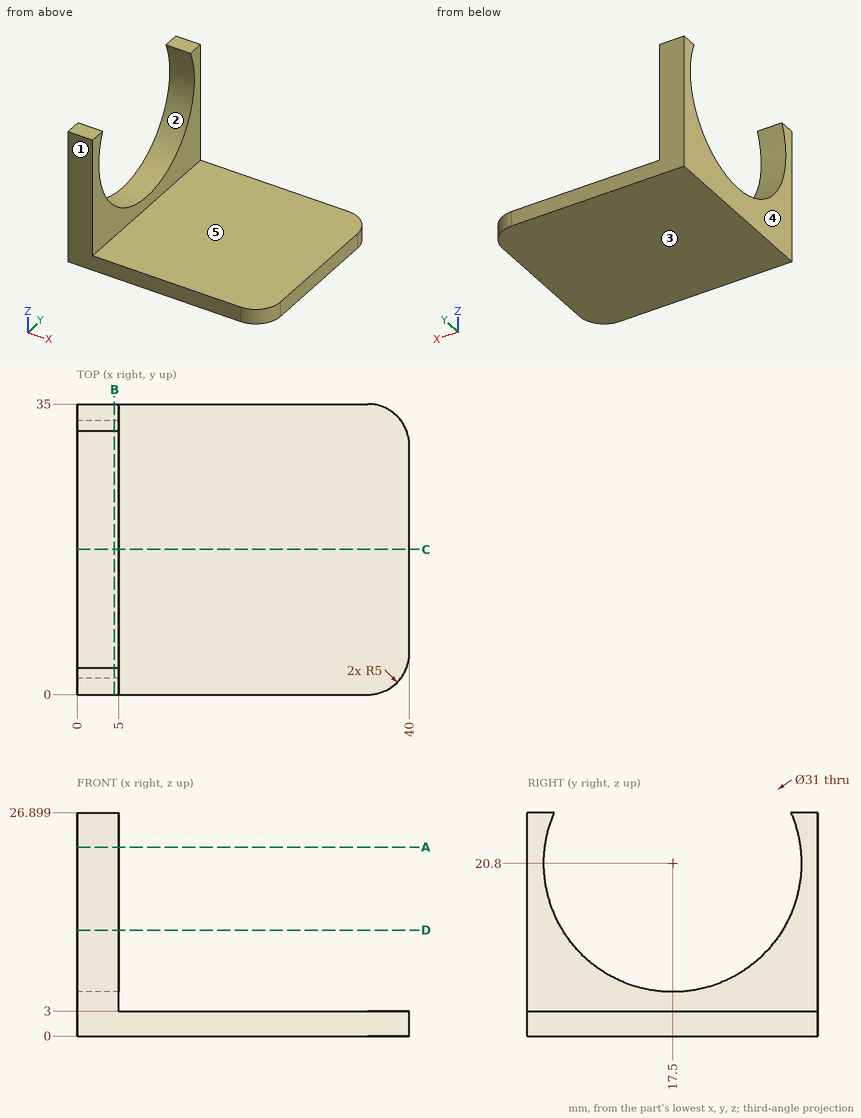
Design review of the part shown in the three views and the two pictorial views. Dimensions are in mm from the part's minimum x, y and z. A direction names the side the tool comes from. Give positions to 0.01 mm unless a question says otherwise; leave off trailing zeros. Loops run counter-clockwise (first coordinate to the right, second up) from the corner with the lowest first, then second, coordinate; pieces in that order, holes last. Notation, with made-up numbers: (36.5, 69.25) -> (56.5, 69.25) arc R20 cw to (56.5, 106.25) -> close; hole circle Ø8 at (-28, 51.25). An arc over 180 degrees is marked (long way). One line per item, written item: value.
Q1. We need section C-C on y = 17.5. Give the boundary of the cut face in (x, z).
Numbers:
outline: (0, 0) -> (40, 0) -> (40, 3) -> (5, 3) -> (5, 5.3) -> (0, 5.3) -> close
Q2. We need section B-B on x = 4.5. Give the boundary of the cut face in (y, z), and give its area (3 significant figures).
Numbers:
outline: (0, 0) -> (35, 0) -> (35, 26.9) -> (31.75, 26.9) arc R15.5 cw (long way) to (3.25, 26.9) -> (0, 26.9) -> close
area: 380 mm^2
Q3. For L1, parallel to Z at x = 37, y = 31.5; L2, parallel to Z at x = 2, y = 17; L3, parallel to X at y = 3, z = 14, list the stretches that pass through material, from the lowest coordinate up.
Numbers:
L1: z = 0 to 3
L2: z = 0 to 5.31
L3: x = 0 to 5
Q4. For pin 1 Ø3 at (x, y) = (25, 21) entering from +Z; pin 2 Ø3 at (y, z) = (4, 3) entering from -X, all flat-tipped, find the tip position at first contact; note any pin that passes through.
Numbers:
pin 1: stops at z = 3
pin 2: stops at x = 0
Q5. Machinability: for the marked faces 4 and 5, which of the approach directions +Z, -Z, +X, -X, +Y, -Y give a long, thin tool a straight path to every point of the face, cutting with its end or side? Answer none if there is none.
Numbers:
face 4: +Z, -Z, -X, +Y, -Y
face 5: +Z, +X, +Y, -Y
Q6. We need section A-A on z = 22.75. Give the boundary of the cut face in (x, y).
Numbers:
outline: (0, 0) -> (5, 0) -> (5, 2.12) -> (0, 2.12) -> close; (0, 32.88) -> (5, 32.88) -> (5, 35) -> (0, 35) -> close
Q7. Draft analysis for pull direction Z (two halves, no side actions). For the marked faces 1, 2 and 3, state which applies: pulls with the +Z half, pulls with the -Z half, needs draft (parallel to the pull), parting line crosses it, or undercut.
Numbers:
face 1: needs draft
face 2: undercut
face 3: pulls with the -Z half
Q8. We need section D-D on z = 12.75. Give the boundary of the cut face in (x, y) (1 decimal).
Numbers:
outline: (0, 0) -> (5, 0) -> (5, 4.3) -> (0, 4.3) -> close; (0, 30.7) -> (5, 30.7) -> (5, 35) -> (0, 35) -> close
